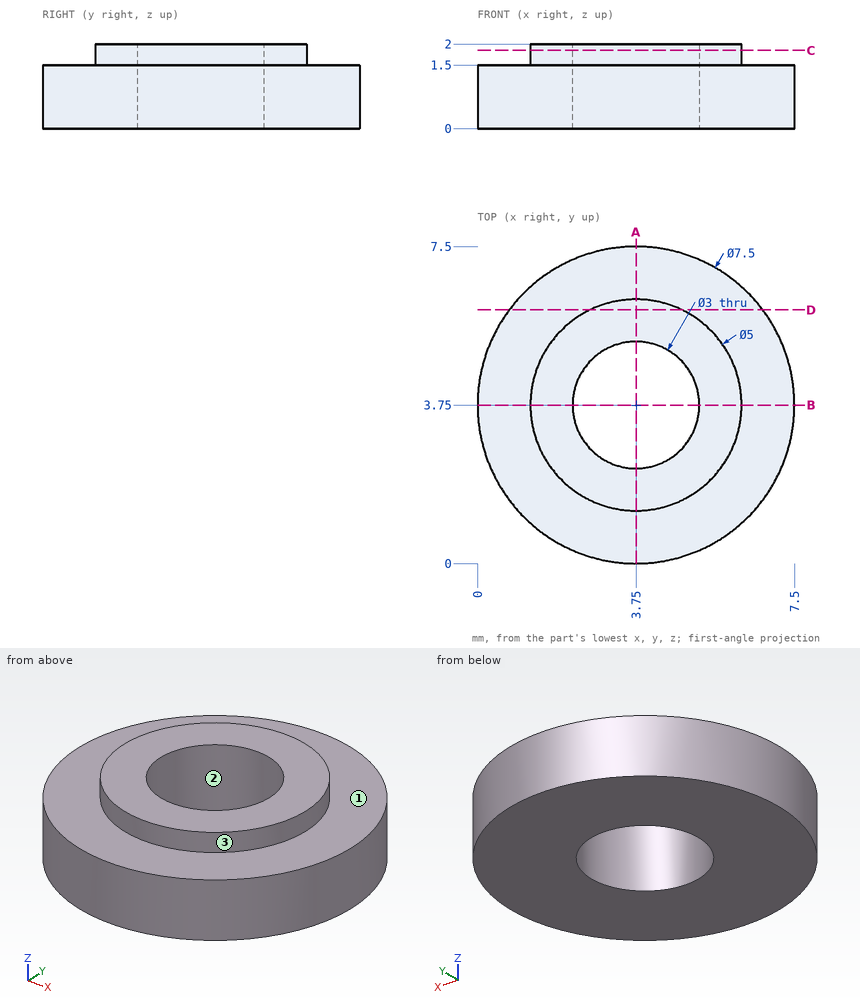
Job drawing, mm, ordinate dimensions from the low corner. One solid piece. Coordinates: 2 decimals unless noted, no trailing zeros. Order: outer loops, then holes, each group sorted by start corner. A loop starts at its lowest first (then second) coordinate and runs counter-clockwise, first axis right, second up. Notation, with made-up numbers: (82, 78.25) -> (103, 78.25) arc R8 cw to (103, 88.25) -> close; hole circle Ø2 at (85.25, -33). An arc over 180 degrees is marked (long way). Put each result on its own line as item: value. Start each with the question number.
(1) Probe line 1 along Y through (x, z) = (3.75, 0.55); line 2 along Z through (x, y) = (1, 4); line 3 along Y through (x, z) = (2.75, 0.85). List the from-to ranges inside material, lowest first. Write a range as [from, to].
(2) Band-saw the part on D-D (y = 6). Give the cut face in (x, z), then the cut area to 3 significant figures.
(3) Pin check, flat tips, straight feed: pin 1 Ø4 at (x, y) = (3.75, 3.75) entering from +Z; pin 2 Ø1 at (x, z) = (2.5, 0.5) entering from +Y; pin 3 Ø1 at (y, z) = (3, 0.5) entering from -X. Stop position of each tip, or through.
(4) Mould opens along Y. For the marked faces 1, 2 and 3 say: pulls with the +Y half, pulls with the -Y half, needs draft (parallel to the pull), parting line crosses it, or undercut.
(5) Band-saw the part on A-A (x = 3.75). Give the cut face in (y, z), then the cut area to 3 significant figures.
(6) Band-saw the part on C-C (z = 1.85). Give the cut face in (x, y), then the cut area to 3 significant figures.
Determined:
1. line 1: y = [0, 2.25], [5.25, 7.5]
1. line 2: z = [0, 1.5]
1. line 3: y = [0.14, 2.63], [4.87, 7.36]
2. outline: (0.75, 0) -> (6.75, 0) -> (6.75, 1.5) -> (4.84, 1.5) -> (4.84, 2) -> (2.66, 2) -> (2.66, 1.5) -> (0.75, 1.5) -> close
2. area: 10.1 mm²
3. pin 1: stops at z = 2
3. pin 2: stops at y = 7.42
3. pin 3: stops at x = 0.01
4. face 1: needs draft
4. face 2: undercut
4. face 3: parting line crosses it
5. outline: (0, 0) -> (2.25, 0) -> (2.25, 2) -> (1.25, 2) -> (1.25, 1.5) -> (0, 1.5) -> close; (5.25, 0) -> (7.5, 0) -> (7.5, 1.5) -> (6.25, 1.5) -> (6.25, 2) -> (5.25, 2) -> close
5. area: 7.75 mm²
6. outline: circle Ø5 at (3.75, 3.75); hole circle Ø3 at (3.75, 3.75)
6. area: 12.6 mm²
